Design review of the part built by this model. Coordinates are the model's own, in mm. A direction names the side the tool comes from. Give positions to 0.01 mm unless a question says otherwise; leave off trailing zeros. Loops run counter-clockwise (first coordinate to the right, second up) from the corner with the lowest first, then second, coordinate; pieces in that order, holes last. Notation, with made-up numbers: (23, 84) -> (32, 84) arc R8 cw to (32, 94) -> close; hole circle Ø6 at (70.25, 8). An arc over 180 degrees is marked (long way). Answer as CSV lines item,"result".
from build123d import *

# Parameters (mm, degrees)
ESQUISSE1_W             = 150
ESQUISSE1_H             = 14
BOSS_EXTRU_1_DEPTH      = 100
BOSS_EXTRU_2_DEPTH      = 25
BOSS_EXTRU_2_DEPTH_BACK = 125
ESQUISSE3_W             = 40
ESQUISSE3_H             = 56
COQUE1_T                = -4
ESQUISSE2_R             = 1.25
ENL_V_MAT_EXTRU_1_DEPTH = 150.916643506


with BuildPart() as part:
    # Esquisse1 → Boss.-Extru.1 (new body)
    with BuildSketch(Plane(origin=(0, 0, 0), x_dir=(1, 0, 0), z_dir=(0, 1, 0))):
        Rectangle(ESQUISSE1_W, ESQUISSE1_H)
        Polygon((66.917096231, 21), (75, 7), (-75, 7), (-66.917096231, 21), align=None)
    boss_extru_1 = extrude(amount=BOSS_EXTRU_1_DEPTH)

    # Symétrie1: Boss.-Extru.1 across plane
    add(boss_extru_1.mirror(Plane(origin=(0, 100, 7), x_dir=(1, 0, 0), z_dir=(0, 0, -1))))

    # Esquisse3 → Boss.-Extru.2 (add, two sides: drawn at the far end of the back side and taken through both)
    with BuildSketch(Plane.XZ.offset(-BOSS_EXTRU_2_DEPTH_BACK)):
        with Locations((0, 7)):
            Rectangle(ESQUISSE3_W, ESQUISSE3_H)
    extrude(amount=BOSS_EXTRU_2_DEPTH + BOSS_EXTRU_2_DEPTH_BACK)

    # Coque1
    coque1_openings = [part.faces().sort_by_distance(p)[0] for p in [
        (0, 50, -21),
    ]]
    offset(amount=COQUE1_T, openings=coque1_openings, kind=Kind.INTERSECTION)

    # Esquisse2 → Enlèv. mat.-Extru.1 (cut, through all)
    with BuildSketch(Plane(origin=(0, 100, 0), x_dir=(1, 0, 0), z_dir=(0, 1, 0))):
        with Locations(Location((45, -26.45, 0), (0, 0, 270))):
            Circle(ESQUISSE2_R)
        with Locations(Location((61.844194104, 2.725, 0), (0, 0, 270))):
            Circle(ESQUISSE2_R)
        with Locations(Location((28.155805896, 2.725, 0), (0, 0, 270))):
            Circle(ESQUISSE2_R)
    enl_v_mat_extru_1 = extrude(amount=-ENL_V_MAT_EXTRU_1_DEPTH, mode=Mode.SUBTRACT)

    # Symétrie2: Enlèv. mat.-Extru.1 across plane
    add(enl_v_mat_extru_1.mirror(Plane(origin=(0, 0, 0), x_dir=(0, 0, 1), z_dir=(1, 0, 0))), mode=Mode.SUBTRACT)


solid = part.part
Q1. To check wall thickness, follow probe 1 along Y at (x, z) = (10.5, 22.5); probe 2 along Y at (x, z) = (-41.5, 26.5); probe 3 along X at (y, z) = (107, -12). State the ranges of each line that lie inside material, in increasing order. Write a range as from..to.
Filled sheet:
probe 1,"y = -25..-21, 121..125"
probe 2,"y = 0..4, 96..100"
probe 3,"x = -20..-16, 16..20"
Q2. For faces 5 (the flat face through (67.76, 49.36, 25.54)), 6 (the flat face through (47, 100, 7)), 7 (the flat face through (0, -21, 5)), list the 3-axis set-ups (+Z, -Z, +X, -X, +Y, -Y) from which the entire face can be reached by the end or side of a thin tool; tool diameter is ignored.
Filled sheet:
face 5,"none"
face 6,"+Z, -Z, +X, +Y"
face 7,"-Z"
Q3. We need section D-D, the plane y = 68. State the section outline as (x, z) points, and give its area (3 significant figures).
Filled sheet:
outline,"(-75, -7) -> (-66.92, -21) -> (-62.3, -21) -> (-71, -5.93) -> (-71, 19.93) -> (-64.61, 31) -> (64.61, 31) -> (71, 19.93) -> (71, -5.93) -> (62.3, -21) -> (66.92, -21) -> (75, -7) -> (75, 21) -> (66.92, 35) -> (-66.92, 35) -> (-75, 21) -> close"
area,"992 mm^2"
Q4. We need section B-B, the plane y = 102. State the section outline as (x, z) points, and give its area (3 significant figures).
Filled sheet:
outline,"(-20, -21) -> (-16, -21) -> (-16, 31) -> (16, 31) -> (16, -21) -> (20, -21) -> (20, 35) -> (-20, 35) -> close"
area,"576 mm^2"
Q5. The part is to be moulded in two halves that separate along Z. For faces 1 (the flat face through (0, -25, 7)), 2 (the flat face through (-71.015, 49.3, -13.902)), 3 (the flat face through (-66.71, 49.36, -13.36)), 4 (the flat face through (-67.849, 49.356, 25.387)), say which applies: pulls with the +Z half, pulls with the -Z half, needs draft (parallel to the pull), parting line crosses it, or undercut.
Filled sheet:
face 1,"needs draft"
face 2,"pulls with the -Z half"
face 3,"undercut"
face 4,"undercut"
Q6. We need section A-A, the plane x = 52. State the section outline as (y, z) points.
Filled sheet:
outline,"(0, -21) -> (4, -21) -> (4, 31) -> (96, 31) -> (96, -21) -> (100, -21) -> (100, 35) -> (0, 35) -> close"
Q7. We need section C-C, the plane z = -15.5. State the section outline as (x, y) points.
Filled sheet:
outline,"(-70.09, 0) -> (-20, 0) -> (-20, -25) -> (20, -25) -> (20, 0) -> (70.09, 0) -> (70.09, 100) -> (20, 100) -> (20, 125) -> (-20, 125) -> (-20, 100) -> (-70.09, 100) -> close; hole (-65.47, 4) -> (-16, 4) -> (-16, -21) -> (16, -21) -> (16, 4) -> (65.47, 4) -> (65.47, 96) -> (16, 96) -> (16, 121) -> (-16, 121) -> (-16, 96) -> (-65.47, 96) -> close"
Q8. Clearance check with flat-ended pins moving along their axes: pin 1 Ø16.5 at (x, z) = (-57.5, 19) entering from +Y; pin 2 Ø4 at (x, z) = (45, 26.45) entering from -Y; pin 3 Ø1.5 at (y, z) = (-5, -11.5) entering from -X. State where each tip first meets the part, or that it passes through.
Filled sheet:
pin 1,"stops at y = 100"
pin 2,"stops at y = 0"
pin 3,"stops at x = -20"
